```python
from build123d import *

# Parameters (mm, degrees)
SALIENTE_EXTRUIR2_DEPTH = 8
CROQUIS3_R              = 2.5
CORTAR_EXTRUIR1_DEPTH   = 31
CROQUIS4_W              = 0.1
CROQUIS4_H              = 0.1
SALIENTE_EXTRUIR3_DEPTH = 0.1
CROQUIS5_W              = 1
CROQUIS5_H              = 0.8740111
CORTAR_EXTRUIR2_DEPTH   = 10
CROQUIS6_W              = 1
CROQUIS6_H              = 1
CORTAR_EXTRUIR3_DEPTH   = 10
CROQUIS8_W              = 1
CROQUIS8_H              = 1
CORTAR_EXTRUIR4_DEPTH   = 10


with BuildPart() as part:
    # Croquis1 → Saliente-Extruir2 (new body)
    with BuildSketch(Plane(origin=(0, 0, 0), x_dir=(1, 0, 0), z_dir=(0, 1, 0))):
        Polygon((71.602540378, 0), (86.602540378, 25.980762114), (15, 150), (-15, 150), (-86.602540378, 25.980762114), (-71.602540378, 0), align=None)
    extrude(amount=SALIENTE_EXTRUIR2_DEPTH)

    # Croquis3 → Cortar-Extruir1 (cut)
    with BuildSketch(Plane(origin=(0, 8, 0), x_dir=(1, 0, 0), z_dir=(0, 1, 0))):
        with Locations(Location((-16, 129, 0), (0, 0, 270))):
            Circle(CROQUIS3_R)
        with Locations(Location((16, 129, 0), (0, 0, 270))):
            Circle(CROQUIS3_R)
        with Locations(Location((-52.916006899, 9.633974596, 0), (0, 0, 270))):
            Circle(CROQUIS3_R)
        with Locations(Location((-68.916006899, 37.346787517, 0), (0, 0, 270))):
            Circle(CROQUIS3_R)
        with Locations(Location((52.916006899, 9.633974596, 0), (0, 0, 270))):
            Circle(CROQUIS3_R)
        with Locations(Location((68.916006899, 37.346787517, 0), (0, 0, 270))):
            Circle(CROQUIS3_R)
    extrude(amount=-CORTAR_EXTRUIR1_DEPTH, mode=Mode.SUBTRACT)

    # Croquis4 → Saliente-Extruir3 (add)
    with BuildSketch(Plane(origin=(0, 8, 0), x_dir=(1, 0, 0), z_dir=(0, 1, 0))):
        with Locations((0, 150)):
            Rectangle(CROQUIS4_W, CROQUIS4_H)
    extrude(amount=SALIENTE_EXTRUIR3_DEPTH)

    # Croquis5 → Cortar-Extruir2 (cut)
    with BuildSketch(Plane(origin=(-53.701905284, 0, 31.004809472), x_dir=(0.5000000000000006, 0, 0.8660254037844384), z_dir=(-0.8660254037844384, 0, 0.5000000000000006))):
        with Locations((-50.801270189, 0)):
            Rectangle(CROQUIS5_W, CROQUIS5_H)
    extrude(amount=-CORTAR_EXTRUIR2_DEPTH, mode=Mode.SUBTRACT)

    # Croquis6 → Cortar-Extruir3 (cut)
    with BuildSketch(Plane(origin=(53.701905284, 0, 31.004809472), x_dir=(0.4999999999999996, 0, -0.8660254037844389), z_dir=(0.8660254037844389, 0, 0.4999999999999996))):
        with Locations((50.801270189, 0)):
            Rectangle(CROQUIS6_W, CROQUIS6_H)
    extrude(amount=-CORTAR_EXTRUIR3_DEPTH, mode=Mode.SUBTRACT)

    # Croquis8 → Cortar-Extruir4 (cut)
    with BuildSketch(Plane(origin=(0, 0, -150), x_dir=(-1, 0, 0), z_dir=(0, 0, -1))):
        Rectangle(CROQUIS8_W, CROQUIS8_H)
    extrude(amount=-CORTAR_EXTRUIR4_DEPTH, mode=Mode.SUBTRACT)


solid = part.part
```
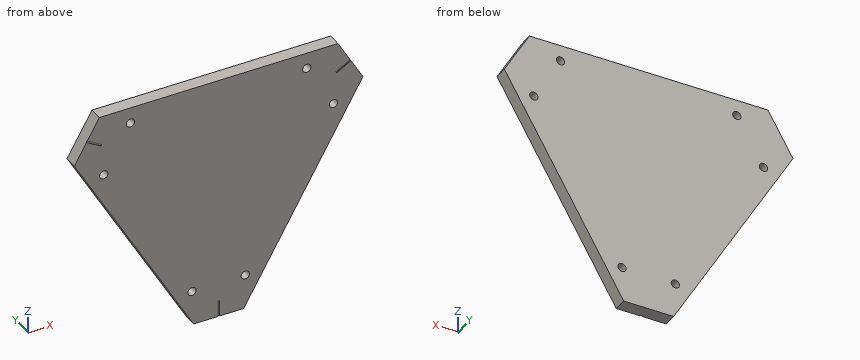
Check sheet for the modelled part. Datum: model origin and axes. Units: mm. Coordinates: 2 decimals unless noted, no trailing zeros. Write each loop counter-clockwise with the first axis right and the second up, starting at its lowest first coordinate (ties: lowest second). Pieces come first, ordered by that corner, then holes. Notation, with made-up numbers: (85.5, -23) -> (109.5, -23) arc R9 ccw to (109.5, -14) -> close; hole circle Ø7 at (85, -35.5). An arc over 180 degrees is marked (long way). Use a Markdown table: item, result.
1. Sectioned sample at A-A (z = -129). Enter the section's corners in (x, y), plus the area to 3 significant figures.
Reported:
| item | result |
|---|---|
| outline | (-27.12, 0) -> (-18.5, 0) -> (-18.5, 8) -> (-27.12, 8) -> close; (-13.5, 0) -> (13.5, 0) -> (13.5, 8) -> (-13.5, 8) -> close; (18.5, 0) -> (27.12, 0) -> (27.12, 8) -> (18.5, 8) -> close |
| area | 354 mm2 |
2. Sectioned sample at C-C (x = 28.5). Enter the section's corners in (y, z).
Reported:
| item | result |
|---|---|
| outline | (0, -126.62) -> (8, -126.62) -> (8, 0) -> (0, 0) -> close |
3. Scan lines: line 1 along X through (y, z) = (2, -127); line 2 along X through (y, z) = (4, -129); line 3 along Y through (x, z) = (4, -23). Record each from-to range of solid material in increasing order.
Reported:
| item | result |
|---|---|
| line 1 | x = -28.28 to -17.5, -14.5 to 14.5, 17.5 to 28.28 |
| line 2 | x = -27.12 to -18.5, -13.5 to 13.5, 18.5 to 27.12 |
| line 3 | y = 0 to 8 |
4. Go/stop test with flat-tipped pins: pin 1 Ø4.5 at (x, z) = (-52.92, -9.63) entering from +Y; pin 2 Ø4 at (y, z) = (3, -76) entering from +X; pin 3 Ø4 at (y, z) = (5.5, -56) entering from +X; pin 4 Ø1 at (x, y) = (24, 1.5) entering from -Z. Record where each tip stops, or that it passes through.
Reported:
| item | result |
|---|---|
| pin 1 | passes through |
| pin 2 | stops at x = 58.88 |
| pin 3 | stops at x = 70.43 |
| pin 4 | stops at z = -135.28 |
5. Sectioned sample at B-B (y = 5.75). Enter the section's corners in (x, z).
Reported:
| item | result |
|---|---|
| outline | (-86.6, -25.98) -> (-15, -150) -> (15, -150) -> (86.6, -25.98) -> (71.6, 0) -> (-71.6, 0) -> close; hole circle Ø5 at (-68.92, -37.35); hole circle Ø5 at (-52.92, -9.63); hole circle Ø5 at (-16, -129); hole circle Ø5 at (16, -129); hole circle Ø5 at (52.92, -9.63); hole circle Ø5 at (68.92, -37.35) |
6. Sectioned sample at D-D (z = -98). Enter the section's corners in (x, y), plus the area to 3 significant figures.
Reported:
| item | result |
|---|---|
| outline | (-45.02, 0) -> (45.02, 0) -> (45.02, 8) -> (-45.02, 8) -> close |
| area | 720 mm2 |
